```python
from build123d import *

# Parameters (mm, degrees)
SALIENTE_EXTRUIR1_DEPTH    = 170
CROQUIS2_W                 = 8
CROQUIS2_H                 = 27
CORTAR_EXTRUIR1_DEPTH      = 1
CORTAR_EXTRUIR1_DEPTH_BACK = 16
CROQUIS3_W                 = 38.06511858
CROQUIS3_H                 = 175.826127046
CORTAR_EXTRUIR2_DEPTH      = 1
CORTAR_EXTRUIR2_DEPTH_BACK = 16
CROQUIS4_W                 = 35.532251822
CROQUIS4_H                 = 7.536766594
CORTAR_EXTRUIR3_DEPTH      = 1
CORTAR_EXTRUIR3_DEPTH_BACK = 171


with BuildPart() as part:
    # Croquis1 → Saliente-Extruir1 (new body)
    with BuildSketch(Plane(origin=(0, 0, 0), x_dir=(1, 0, 0), z_dir=(0, 1, 0))):
        Polygon((0, 0), (17.50080029, 15), (60, 15), (60, 0), align=None)
    extrude(amount=SALIENTE_EXTRUIR1_DEPTH)

    # Croquis2 → Cortar-Extruir1 (cut, two sides)
    with BuildSketch(Plane(origin=(0, 0, -15), x_dir=(-1, 0, 0), z_dir=(0, 0, -1))) as cortar_extruir1_sk:
        with Locations((-56, 13.5)):
            Rectangle(CROQUIS2_W, CROQUIS2_H)
        with Locations((-56, 156.5)):
            Rectangle(CROQUIS2_W, CROQUIS2_H)
    extrude(amount=CORTAR_EXTRUIR1_DEPTH, mode=Mode.SUBTRACT)
    extrude(cortar_extruir1_sk.sketch, amount=-CORTAR_EXTRUIR1_DEPTH_BACK, mode=Mode.SUBTRACT)

    # Croquis3 → Cortar-Extruir2 (cut, two sides)
    with BuildSketch(Plane(origin=(0, 0, -15), x_dir=(-1, 0, 0), z_dir=(0, 0, -1))) as cortar_extruir2_sk:
        with Locations((-65.03255929, 82.086936477)):
            Rectangle(CROQUIS3_W, CROQUIS3_H)
    extrude(amount=CORTAR_EXTRUIR2_DEPTH, mode=Mode.SUBTRACT)
    extrude(cortar_extruir2_sk.sketch, amount=-CORTAR_EXTRUIR2_DEPTH_BACK, mode=Mode.SUBTRACT)

    # Croquis4 → Cortar-Extruir3 (cut, two sides)
    with BuildSketch(Plane.XZ) as cortar_extruir3_sk:
        with Locations((28.233874089, -16.468383297)):
            Rectangle(CROQUIS4_W, CROQUIS4_H)
    extrude(amount=CORTAR_EXTRUIR3_DEPTH, mode=Mode.SUBTRACT)
    extrude(cortar_extruir3_sk.sketch, amount=-CORTAR_EXTRUIR3_DEPTH_BACK, mode=Mode.SUBTRACT)


solid = part.part
```
Geometry check sheet. Reference: the model listing, model coordinates, mm. Coordinates: 2 decimals unless noted, no trailing zeros. Order: outer loops, then holes, each group sorted by start corner. A loop starts at its lowest first (then second) coordinate and runs counter-clockwise, first axis right, second up. Notation, with made-up numbers: (74, -4.75) - (119, -4.75) arc R11 ccw to (119, 14.25) - close; hole circle Ø2 at (43.25, 54.5). An arc over 180 degrees is marked (long way). Use one line per item in the form item = value.
1. Scan lines: line 1 (Z direction, x = 3.5, y = 153.5); line 2 (X direction, y = 38, z = -12); line 3 (X direction, y = 15.5, z = -3). Record each from-to range of solid material in increasing order.
Here are the results:
line_1 = -3 to 0
line_2 = 14 to 46
line_3 = 3.5 to 46
2. Section check A-A (y = 32). Record the boundary of the cut face in (x, z).
Here are the results:
outline = (0, 0) - (14.82, -12.7) - (46, -12.7) - (46, 0) - close
3. Section check B-B (z = -9.25). Record the boundary of the cut face in (x, y).
Here are the results:
outline = (10.79, 0) - (46, 0) - (46, 170) - (10.79, 170) - close
4. Gauge pin test, flat end, axial feed: pin 1 (1.5 mm diameter, centred on x = 36, y = 88.5, fed in from +Z). Record the tip position at first contact, or that the pin passes through.
Here are the results:
pin_1 = 0
